Could you check a few things on this model? Use its own coordinates, in mm. A direction names the side the tool comes from. Coordinates: 2 decimals unless noted, no trailing zeros. Loops run counter-clockwise (first coordinate to the right, second up) from the corner with the lowest first, then second, coordinate; pieces in that order, holes last.
1) Imagine slicing it at C-C on z = 3. Please give me the cut outline in (x, y).
2) For faces 4 (the face through (-21.59, -8, 6)), 5 (the face through (28, -17.78, 6)), 6 (the face through (-14, 4, 0.254)), which set-ups out of +Z, -Z, +X, -X, +Y, -Y let a thin tool reach every point of the face, with its end or its side?
3) Thinking about a two-plate mould opening in Y: for faces 1 (the face through (6.14, -11.32, 0)), 2 (the face through (22.4, -17.1, 6.3)), 3 (the face through (-14, 4, 12.446)), which applies, released by +Y, released by -Y, zero draft, split by the parting line, or undercut?
4) Will these pins go through, and if not, where does the flat tip stop? P1, Ø6.5, axis at y = -8, z = 9.5, coming from the -X side; P2, Ø2.5, axis at x = 29.5, z = 4, coming from the +Y side; P3, Ø5, axis at y = 8, z = 5.5, coming from the +X side.
5) Imagine slicing it at B-B on y = 3. Please give me the cut outline in (x, z).
6) If I drill on line 1 along Y through (x, z) = (0, 0.1); line 2 along Y through (x, z) = (0, 6.75); line 3 along Y through (x, z) = (27.5, 5.5), over which ranges is the centre line in solid material (lowest first)?
7) Imagine slicing it at A-A on x = 0. Please give me the cut outline in (y, z).
8) Imagine slicing it at D-D on x = -15. Please give me the cut outline in (y, z).
```python
from build123d import *

# Parameters (mm, degrees)
SKETCH1_R           = 17.78
SKETCH1_R_2         = 12.7
BOSS_EXTRUDE1_DEPTH = 12.7
SKETCH2_R           = 16.51
SKETCH2_R_2         = 13.97
CUT_EXTRUDE1_DEPTH  = 0.254
SKETCH3_R           = 17.78
BOSS_EXTRUDE3_DEPTH = 12.7


with BuildPart() as part:
    # Sketch1 → Boss-Extrude1 (new body)
    with BuildSketch(Plane.XY):
        Circle(SKETCH1_R)
        Circle(SKETCH1_R_2, mode=Mode.SUBTRACT)
    extrude(amount=BOSS_EXTRUDE1_DEPTH)

    # Sketch2 → Cut-Extrude1 (cut)
    with BuildSketch(Plane.XY.offset(12.7)):
        Circle(SKETCH2_R)
        Circle(SKETCH2_R_2, mode=Mode.SUBTRACT)
    cut_extrude1 = extrude(amount=-CUT_EXTRUDE1_DEPTH, mode=Mode.SUBTRACT)

    # Mirror1: Cut-Extrude1 across plane
    add(cut_extrude1.mirror(Plane.XY.offset(6.35)), mode=Mode.SUBTRACT)

    # Sketch3 → Boss-Extrude3 (add)
    with BuildSketch(Plane.XY):
        with BuildLine():
            Line((-31.75, -21.59), (31.75, -21.59))
            Line((31.75, -21.59), (31.75, -17.78))
            Line((31.75, -17.78), (24.13, -17.78))
            ThreePointArc((24.13, -17.78), (22.333948776, -17.036051224), (21.59, -15.24))
            Line((21.59, -15.24), (21.59, 0))
            ThreePointArc((21.59, 0), (0, 21.59), (-21.59, 0))
            Line((-21.59, 0), (-21.59, -15.24))
            ThreePointArc((-21.59, -15.24), (-22.333948776, -17.036051224), (-24.13, -17.78))
            Line((-24.13, -17.78), (-31.75, -17.78))
            Line((-31.75, -17.78), (-31.75, -21.59))
        make_face()
        Circle(SKETCH3_R, mode=Mode.SUBTRACT)
    extrude(amount=BOSS_EXTRUDE3_DEPTH)


solid = part.part
```
Filled in:
1. outline: (-31.75, -21.59) - (31.75, -21.59) - (31.75, -17.78) - (24.13, -17.78) arc R2.54 cw to (21.59, -15.24) - (21.59, 0) arc R21.59 ccw to (-21.59, 0) - (-21.59, -15.24) arc R2.54 cw to (-24.13, -17.78) - (-31.75, -17.78) - close; hole circle Ø25.4 at (0, 0)
2. face 4: +Z, -Z, -X, +Y
2. face 5: +Z, -Z, +X, +Y
2. face 6: -Z
3. face 1: zero draft
3. face 2: released by +Y
3. face 3: undercut
4. P1: stops at x = -21.59
4. P2: stops at y = -17.78
4. P3: stops at x = 20.88
5. outline: (-21.38, 0) - (-16.24, 0) - (-16.24, 0.25) - (-13.64, 0.25) - (-13.64, 0) - (-12.34, 0) - (-12.34, 12.7) - (-13.64, 12.7) - (-13.64, 12.45) - (-16.24, 12.45) - (-16.24, 12.7) - (-21.38, 12.7) - close; (12.34, 0) - (13.64, 0) - (13.64, 0.25) - (16.24, 0.25) - (16.24, 0) - (21.38, 0) - (21.38, 12.7) - (16.24, 12.7) - (16.24, 12.45) - (13.64, 12.45) - (13.64, 12.7) - (12.34, 12.7) - close
6. line 1: y = -21.59 to -16.51, -13.97 to -12.7, 12.7 to 13.97, 16.51 to 21.59
6. line 2: y = -21.59 to -12.7, 12.7 to 21.59
6. line 3: y = -21.59 to -17.78
7. outline: (-21.59, 0) - (-16.51, 0) - (-16.51, 0.25) - (-13.97, 0.25) - (-13.97, 0) - (-12.7, 0) - (-12.7, 12.7) - (-13.97, 12.7) - (-13.97, 12.45) - (-16.51, 12.45) - (-16.51, 12.7) - (-21.59, 12.7) - close; (12.7, 0) - (13.97, 0) - (13.97, 0.25) - (16.51, 0.25) - (16.51, 0) - (21.59, 0) - (21.59, 12.7) - (16.51, 12.7) - (16.51, 12.45) - (13.97, 12.45) - (13.97, 12.7) - (12.7, 12.7) - close
8. outline: (-21.59, 0) - (-6.9, 0) - (-6.9, 0.25) - (6.9, 0.25) - (6.9, 0) - (15.53, 0) - (15.53, 12.7) - (6.9, 12.7) - (6.9, 12.45) - (-6.9, 12.45) - (-6.9, 12.7) - (-21.59, 12.7) - close
